Verification items for the finished model (mm, model axes). A direction names the side the tool comes from. Coordinates: 2 decimals unless noted, no trailing zeros. Loops run counter-clockwise (first coordinate to the right, second up) from the corner with the lowest first, then second, coordinate; pieces in that order, holes last.
Q1. Mould release check, pull along Y, two halves, no side actions. Record for faces 1 (the face through (189, 1, 3)), 2 (the face through (162.933, 6.131, 2.717)), 3 (the face through (161.9, 5.9, 1.5)), 4 (the face through (216.133, 6.892, 2.717)): +Y half, -Y half, draft (parallel to the pull), parting line (faces both ways), or undercut.
Q2. Sectioned sample at C-C (x = 180). Enter the section's corners in (y, z).
Q3. Access from +Z, -Z, +X, -X, +Y, -Y to the whole of each face (thin tool, end or side, straight path). Record for faces 5 (the face through (189.2, 2, 1.5)), 6 (the face through (217.3, 5.9, 1.5)), 7 (the face through (189.2, 10, 1.5)), 8 (the face through (189, 6, 4.552)).
Q4. Go/stop test with flat-tipped pins: P1, Ø0.9, axis at x = 177.5, z = 1.5, coming from the -Y side; P2, Ø0.9, axis at y = 5, z = 1.5, coming from the +X side; P3, Ø5.5, axis at x = 165.9, y = 6, coming from the -Z side. Record where each tip stops, or that it passes through.
Q5. Sectioned sample at A-A (x = 165.9). Enter the section's corners in (y, z), then the cut area to 3 significant figures.
Q6. Sectioned sample at D-D (y = 8.25). Enter the section's corners in (x, z), then the cut area to 3 significant figures.
Q7. Sectioned sample at B-B (y = 6). Enter the section's corners in (x, z).
Q8. Material ranges on probe 1 along Y at (x, z) = (213.3, 3.3); probe 2 along X at (y, z) = (8.25, 1.5); probe 3 along X at (y, z) = (5, 2.3), recorded low to high.
```python
from build123d import *

# Parameters (mm, degrees)
SKETCH1_W           = 55.4
SKETCH1_H           = 8
SKETCH1_R           = 2.97
BOSS_EXTRUDE1_DEPTH = 1.12
SKETCH2_W           = 57.4
SKETCH2_H           = 10
SKETCH2_R           = 2.97
BOSS_EXTRUDE2_DEPTH = 2.5


with BuildPart() as part:
    # Sketch1 → Boss-Extrude1 (new body)
    with BuildSketch(Plane.XY.offset(0.931976945)):
        with Locations((189.6, 6)):
            Rectangle(SKETCH1_W, SKETCH1_H)
        with Locations((165.9, 6)):
            Circle(SKETCH1_R, mode=Mode.SUBTRACT)
        with Locations((213.3, 6)):
            Circle(SKETCH1_R, mode=Mode.SUBTRACT)
    extrude(amount=BOSS_EXTRUDE1_DEPTH)

    # Sketch2 → Boss-Extrude2 (add)
    with BuildSketch(Plane.XY.offset(2.051976945)):
        with Locations((189.6, 6)):
            Rectangle(SKETCH2_W, SKETCH2_H)
        with Locations((213.3, 6)):
            Circle(SKETCH2_R, mode=Mode.SUBTRACT)
        with Locations((165.9, 6)):
            Circle(SKETCH2_R, mode=Mode.SUBTRACT)
    extrude(amount=BOSS_EXTRUDE2_DEPTH)


solid = part.part
```
Geometry check:
1. face 1: -Y half
1. face 2: undercut
1. face 3: draft
1. face 4: undercut
2. outline: (1, 2.05) - (2, 2.05) - (2, 0.93) - (10, 0.93) - (10, 2.05) - (11, 2.05) - (11, 4.55) - (1, 4.55) - close
3. face 5: -Z, +X, -X, -Y
3. face 6: -Z, +X, +Y, -Y
3. face 7: -Z, +X, -X, +Y
3. face 8: +Z, +X, -X, +Y, -Y
4. P1: stops at y = 2
4. P2: stops at x = 217.3
4. P3: passes through
5. outline: (1, 2.05) - (2, 2.05) - (2, 0.93) - (3.03, 0.93) - (3.03, 4.55) - (1, 4.55) - close; (8.97, 0.93) - (10, 0.93) - (10, 2.05) - (11, 2.05) - (11, 4.55) - (8.97, 4.55) - close
5. area: 12.5 mm2
6. outline: (160.9, 2.05) - (161.9, 2.05) - (161.9, 0.93) - (163.96, 0.93) - (163.96, 4.55) - (160.9, 4.55) - close; (167.84, 0.93) - (211.36, 0.93) - (211.36, 4.55) - (167.84, 4.55) - close; (215.24, 0.93) - (217.3, 0.93) - (217.3, 2.05) - (218.3, 2.05) - (218.3, 4.55) - (215.24, 4.55) - close
6. area: 177 mm2
7. outline: (160.9, 2.05) - (161.9, 2.05) - (161.9, 0.93) - (162.93, 0.93) - (162.93, 4.55) - (160.9, 4.55) - close; (168.87, 0.93) - (210.33, 0.93) - (210.33, 4.55) - (168.87, 4.55) - close; (216.27, 0.93) - (217.3, 0.93) - (217.3, 2.05) - (218.3, 2.05) - (218.3, 4.55) - (216.27, 4.55) - close
8. probe 1: y = 1 to 3.03, 8.97 to 11
8. probe 2: x = 161.9 to 163.96, 167.84 to 211.36, 215.24 to 217.3
8. probe 3: x = 160.9 to 163.1, 168.7 to 210.5, 216.1 to 218.3
